```python
from build123d import *

# Parameters (mm, degrees)
SKETCH_1_R      = 1.65
EXTRUDE_1_DEPTH = 3
EXTRUDE_2_DEPTH = 2.9
CHAMFER_1_SIZE  = 2.9
FILLET_1_R      = 1


with BuildPart() as part:
    # 草图1 → 凸台-拉伸1 (new body)
    with BuildSketch(Plane.XY):
        Polygon((-85.15, 37.05), (-23.614971157, 37.05), (31.485028843, -18.05), (85.15, -18.05), (85.15, -37.05), (23.614971157, -37.05), (-31.485028843, 18.05), (-85.15, 18.05), align=None)
        with Locations((-75.15, 27.55)):
            Circle(SKETCH_1_R, mode=Mode.SUBTRACT)
        with Locations((75.15, -27.55)):
            Circle(SKETCH_1_R, mode=Mode.SUBTRACT)
    extrude(amount=EXTRUDE_1_DEPTH)

    # 草图2 → 凸台-拉伸2 (add)
    with BuildSketch(Plane.XY.offset(3)):
        Polygon((-66.15, 33.95), (-66.15, 21.15), (-30.200966799, 21.15), (24.899033201, -33.95), (66.15, -33.95), (66.15, -21.15), (30.200966799, -21.15), (-24.899033201, 33.95), align=None)
    extrude(amount=EXTRUDE_2_DEPTH)

    # 倒角1
    chamfer_1_edges = [part.edges().sort_by_distance(p)[0] for p in [
        (66.15, -27.55, 5.9),
        (-66.15, 27.55, 5.9),
    ]]
    chamfer(chamfer_1_edges, length=CHAMFER_1_SIZE - 0.0001)  # a hair under: the kernel refuses the full size

    # 圆角1
    fillet_1_edges = [part.edges().sort_by_distance(p)[0] for p in [
        (-23.614971157, 37.05, 1.5),
        (31.485028843, -18.05, 1.5),
        (23.614971157, -37.05, 1.5),
        (-31.485028843, 18.05, 1.5),
        (-24.899033201, 33.95, 4.45),
        (-30.200966799, 21.15, 4.45),
        (24.899033201, -33.95, 4.45),
        (30.200966799, -21.15, 4.45),
    ]]
    fillet(fillet_1_edges, radius=FILLET_1_R)


solid = part.part
```
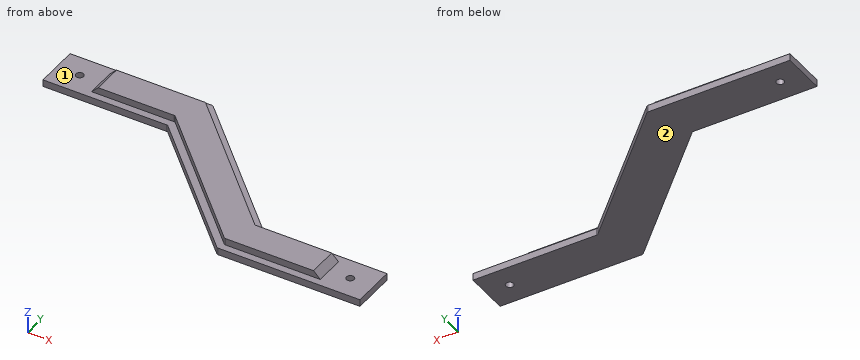
Design review of the part built by this model. Coordinates are the model's own, in mm. Face numbers are marked on the shaded views. A direction names the side the tool comes from. Round coordinates to 2 decimals unless told otherwise and drop trailing zeros. Order: outer loops, then holes, each group sorted by start corner. A loop starts at its lowest first (then second) coordinate and runs counter-clockwise, first axis right, second up. Notation, with made-up numbers: (68, -24) - (93, -24) arc R17 ccw to (93, -16) - close; hole circle Ø6 at (64, -29). An arc over 180 degrees is marked (long way). One line per question, with ' | ' between items.
Item 1: Take a section at D-D, the plane x = 53.5. Write out the cut boundary in (y, z), then the cut area to 3 significant figures.
Checks:
outline: (-37.05, 0) - (-18.05, 0) - (-18.05, 3) - (-21.15, 3) - (-21.15, 5.9) - (-33.95, 5.9) - (-33.95, 3) - (-37.05, 3) - close | area: 94.1 mm²
Item 2: Wall thickness on line 1 (Y direction, x = -75.15, z = 0.8); line 2 (Y direction, x = 41, z = 2.55); line 3 (Y direction, x = -32, z = 3.9): over which ranges is each line inside the solid? List them lowest first. Write a range as [from, to].
Checks:
line 1: [18.05, 25.9], [29.2, 37.05] | line 2: [-37.05, -18.05] | line 3: [21.15, 33.95]
Item 3: For P1, Ø2.5, axis at x = 52, z = 4, coming from the +Y side; P2, Ø3, axis at x = 5, z = 5, coming from the +Y side; P3, Ø2.5, axis at x = -36, z = 5, coming from the +Y side, all flat-tipped, find the tip position at first contact; note any pin that passes through.
Checks:
P1: y = -18.05 | P2: y = 5.55 | P3: y = 33.95
Item 4: Take a section at A-A, the plane x = -75.15. Write out the cut boundary in (y, z), then the cut area to 3 significant figures.
Checks:
outline: (18.05, 0) - (25.9, 0) - (25.9, 3) - (18.05, 3) - close; (29.2, 0) - (37.05, 0) - (37.05, 3) - (29.2, 3) - close | area: 47.1 mm²
Item 5: Take a section at B-B, the plane z = 1.95. Write out the cut boundary in (x, y), then the cut area to 3 significant figures.
Checks:
outline: (-85.15, 18.05) - (-31.9, 18.05) arc R1 cw to (-31.19, 17.76) - (23.32, -36.76) arc R1 ccw to (24.03, -37.05) - (85.15, -37.05) - (85.15, -18.05) - (31.9, -18.05) arc R1 cw to (31.19, -17.76) - (-23.32, 36.76) arc R1 ccw to (-24.03, 37.05) - (-85.15, 37.05) - close; hole circle Ø3.3 at (-75.15, 27.55); hole circle Ø3.3 at (75.15, -27.55) | area: 3,650 mm²
Item 6: Machinability: for the marked faces 1 and 2, which of the approach directions +Z, -Z, +X, -X, +Y, -Y give a long, thin tool a straight path to every point of the face, cutting with its end or side? Answer none if there is none.
Checks:
face 1: +Z | face 2: -Z, +X, -X, +Y, -Y
